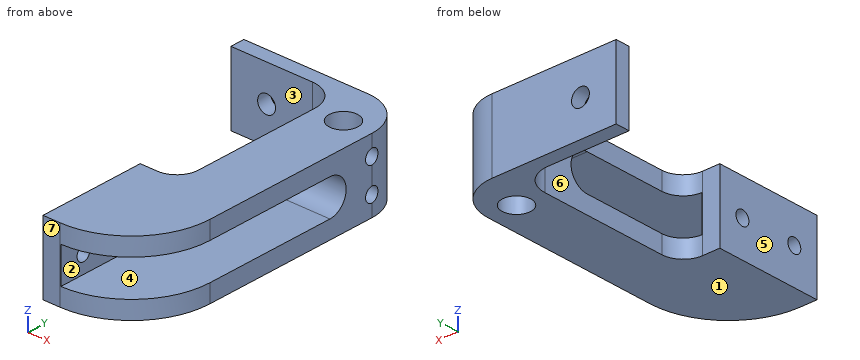
```python
from build123d import *

# Parameters (mm, degrees)
SKETCH1_R           = 4
SKETCH1_R_2         = 2
BOSS_EXTRUDE1_DEPTH = 25
SKETCH2_W           = 20
SKETCH2_H           = 20
CUT_EXTRUDE1_DEPTH  = 30
SKETCH3_R           = 2.5
CUT_EXTRUDE2_DEPTH  = 25
SKETCH6_W           = 100
SKETCH6_H           = 150
CUT_EXTRUDE5_DEPTH  = 5
CUT_EXTRUDE6_DEPTH  = 21.8
SKETCH8_R           = 2
CUT_EXTRUDE7_DEPTH  = 21.8
SKETCH9_R           = 2
CUT_EXTRUDE8_DEPTH  = 6


with BuildPart() as part:
    # Sketch1 → Boss-Extrude1 (new body)
    with BuildSketch(Plane.XY):
        with BuildLine():
            Line((-10, 25), (12.8, 25))
            ThreePointArc((12.8, 25), (18.456854249, 22.656854249), (20.8, 17))
            Line((20.8, 17), (20.8, -19))
            ThreePointArc((20.8, -19), (19.042640687, -23.242640687), (14.8, -25))
            Line((14.8, -25), (-10, -25))
            Line((-10, -25), (-10, -55))
            Line((-10, -55), (14.8, -55))
            ThreePointArc((14.8, -55), (30.356349186, -48.556349186), (36.8, -33))
            Line((36.8, -33), (36.8, 17))
            ThreePointArc((36.8, 17), (33.285281374, 25.485281374), (24.8, 29))
            Line((24.8, 29), (-10, 29))
            Line((-10, 29), (-10, 25))
        make_face()
        with Locations((28.8, 17)):
            Circle(SKETCH1_R, mode=Mode.SUBTRACT)
        with Locations((0, -35)):
            Circle(SKETCH1_R_2, mode=Mode.SUBTRACT)
    extrude(amount=BOSS_EXTRUDE1_DEPTH)

    # Sketch2 → Cut-Extrude1 (cut)
    with BuildSketch(Plane(origin=(0, -25, 0), x_dir=(1, 0, 0), z_dir=(0, 1, 0))):
        with Locations((0, -10)):
            Rectangle(SKETCH2_W, SKETCH2_H)
    extrude(amount=-CUT_EXTRUDE1_DEPTH, mode=Mode.SUBTRACT)

    # Sketch3 → Cut-Extrude2 (cut)
    with BuildSketch(Plane(origin=(0, 29, 0), x_dir=(1, 0, 0), z_dir=(0, 1, 0))):
        with Locations(Location((0, -10, 0), (0, 0, 180))):
            Circle(SKETCH3_R)
    extrude(amount=-CUT_EXTRUDE2_DEPTH, mode=Mode.SUBTRACT)

    # Sketch6 → Cut-Extrude5 (cut)
    with BuildSketch(Plane.XY.offset(25)):
        Rectangle(SKETCH6_W, SKETCH6_H)
    extrude(amount=-CUT_EXTRUDE5_DEPTH, mode=Mode.SUBTRACT)

    # Sketch7 → Cut-Extrude6 (cut)
    with BuildSketch(Plane(origin=(36.8, 0, 0), x_dir=(0, 0, -1), z_dir=(1, 0, 0))):
        with BuildLine():
            Line((-5, 4), (-5, -56))
            ThreePointArc((-5, -56), (-10, -61), (-15, -56))
            Line((-15, -56), (-15, 4))
            ThreePointArc((-15, 4), (-10, 9), (-5, 4))
        make_face()
    extrude(amount=-CUT_EXTRUDE6_DEPTH, mode=Mode.SUBTRACT)

    # Sketch8 → Cut-Extrude7 (cut)
    with BuildSketch(Plane(origin=(15, 0, 0), x_dir=(0, 0, -1), z_dir=(1, 0, 0))):
        with Locations(Location((-10, -31.99666574, 0), (0, 0, 90))):
            Circle(SKETCH8_R)
        with Locations(Location((-10, -47.99909089, 0), (0, 0, 90))):
            Circle(SKETCH8_R)
    extrude(amount=-CUT_EXTRUDE7_DEPTH, mode=Mode.SUBTRACT)

    # Sketch9 → Cut-Extrude8 (cut)
    with BuildSketch(Plane(origin=(36.8, 0, 0), x_dir=(0, 0, -1), z_dir=(1, 0, 0))):
        with Locations(Location((-14.5, 17, 0), (0, 0, 90))):
            Circle(SKETCH9_R)
        with Locations(Location((-5.5, 17, 0), (0, 0, 90))):
            Circle(SKETCH9_R)
    extrude(amount=-CUT_EXTRUDE8_DEPTH, mode=Mode.SUBTRACT)


solid = part.part
```
Input: part model. Units: mm. Frame: model coordinates. Face numbers are marked on the shaded views. A direction names the side the tool comes from. Coordinates: 2 decimals unless noted, no trailing zeros. Loops run counter-clockwise (first coordinate to the right, second up) from the corner with the lowest first, then second, coordinate; pieces in that order, holes last.
Q1. Section C-C, the plane x = 0. Return the cut outline in (y, z), and give its area (3 significant figures).
Results are:
outline: (25, 0) - (29, 0) - (29, 7.5) - (25, 7.5) - close; (25, 12.5) - (29, 12.5) - (29, 20) - (25, 20) - close
area: 60.0 mm2
Q2. Section A-A, the plane y = -32. Return the cut outline in (x, z), and give its area (3 significant figures).
Results are:
outline: (10, 0) - (36.8, 0) - (36.8, 5) - (15, 5) - (15, 8) - (10, 8) - close; (10, 12) - (15, 12) - (15, 15) - (36.8, 15) - (36.8, 20) - (10, 20) - close
area: 298 mm2
Q3. Section D-D, the plane y = -13.5. Return the cut outline in (x, z).
Results are:
outline: (20.8, 0) - (36.8, 0) - (36.8, 5) - (20.8, 5) - close; (20.8, 15) - (36.8, 15) - (36.8, 20) - (20.8, 20) - close
Q4. Line query: line 1 along Z through (x, y) = (34, 17); line 2 along Z through (x, y) = (0, 26.4); line 3 along Z through (x, y) = (23.5, -36). Output: solid intervals per line, ascending.
Results are:
line 1: z = 0 to 3.5, 7.5 to 12.5, 16.5 to 20
line 2: z = 0 to 7.5, 12.5 to 20
line 3: z = 0 to 5, 15 to 20
Q5. Contact query for flat-ended pins moving along their axis: pin 1 (10 mm diameter, centred on y = -38, z = 6, fed in from -X); pin 2 (4.5 mm diameter, centred on y = -48, z = 10, fed in from +X); pin 3 (6 mm diameter, centred on x = 4, z = 12.5, fed in from -Y); pin 4 (5 mm diameter, centred on x = 28.8, y = 17, fed in from -Z). Output: stop coordinate, or through.
Results are:
pin 1: stops at x = 10
pin 2: stops at x = 15
pin 3: stops at y = 25
pin 4: passes through
Q6. Section B-B, the plane x = 14. Return the cut outline in (y, z), and give its area (3 significant figures).
Results are:
outline: (-55, 0) - (-25, 0) - (-25, 20) - (-55, 20) - close; (24.91, 0) - (29, 0) - (29, 20) - (24.91, 20) - close; hole circle Ø4 at (-48, 10); hole circle Ø4 at (-32, 10)
area: 657 mm2
Q7. Set-up query: the marked faces 4, 5, 6 and 7. Return all of +Z, -Z, +X, -X, +Y, -Y with unobstructed straight access to the full face (end or side cutting, diameter ignored); none if empty.
Results are:
face 4: +X, -Y
face 5: +Z, -Z, -X, -Y
face 6: +Z, -Z, -X
face 7: +Z, -Z, +X, -X, -Y
Q8. Mould query, pull axis Z, two halves, no side actions, for the marked faces 1, 2 and 3. Classes: +Z half, -Z half, draft (parallel to the pull), parting line (faces both ways), or undercut.
Results are:
face 1: -Z half
face 2: undercut
face 3: draft
